The listing builds one solid part. Answer for the finished solid, in the listing's coordinates (mm). Give positions to 0.01 mm unless a question says otherwise; leave off trailing zeros. Order: outer loops, then holes, each group sorted by start corner. A loop starts at its lowest first (then second) coordinate and runs counter-clockwise, first axis right, second up. Notation, with made-up numbers: (-27, 42.25) -> (-12, 42.25) arc R23 cw to (-12, 77.25) -> close; hole circle Ø5 at (74.5, 88). An arc over 180 degrees is marked (long way). Answer as a JSON object with one key per item and string values. Group by question number.
Autodesk Inventor part; units mm, degrees
ref_plane "YZ Plane" through (0, 0, 0) normal (1, 0, 0) x (0, 1, 0)
ref_plane "XZ Plane" through (0, 0, 0) normal (0, 1, 0) x (-1, 0, 0)
ref_plane "XY Plane" through (0, 0, 0) normal (0, 0, 1) x (1, 0, 0)
sketch "Sketch1" plane through (0, 0, 0) normal (0, 0, 1) x (1, 0, 0)
  arc A0 (3.9004, -5.517) -> (1.5898, -4.52) centre (1.5898, -7.6958) ccw
  line L0 (6.8514, -8.6465) -> (3.9004, -5.517)
  arc A1 (6.1121, -10.36) -> (6.8514, -8.6465) centre (6.1121, -9.3437) ccw
  line L1 (-6.1121, -10.36) -> (6.1121, -10.36)
  arc A2 (-6.8514, -8.6465) -> (-6.1121, -10.36) centre (-6.1121, -9.3437) ccw
  line L2 (-3.9004, -5.517) -> (-6.8514, -8.6465)
  arc A3 (-1.5898, -4.52) -> (-3.9004, -5.517) centre (-1.5898, -7.6958) ccw
  line L3 (1.5898, -4.52) -> (-1.5898, -4.52)
  arc A4 (-10.36, -6.3382) -> (-8.5738, -7.0738) centre (-9.3466, -6.4137) ccw
  line L4 (-10.36, 6.3382) -> (-10.36, -6.3382)
  arc A5 (-8.5738, 7.0738) -> (-10.36, 6.3382) centre (-9.3466, 6.4137) ccw
  line L5 (-5.4693, 3.7815) -> (-8.5738, 7.0738)
  arc A6 (-4.38, 1.5898) -> (-5.4693, 3.7815) centre (-7.549, 1.3814) ccw
  line L6 (-4.38, -1.5898) -> (-4.38, 1.5898)
  arc A7 (-5.4693, -3.7815) -> (-4.38, -1.5898) centre (-7.549, -1.3814) ccw
  line L7 (-8.5738, -7.0738) -> (-5.4693, -3.7815)
  arc A8 (8.5693, -7.069) -> (10.36, -6.3423) centre (9.3463, -6.4139) ccw
  line L8 (5.2366, -3.5348) -> (8.5693, -7.069)
  arc A9 (4.38, -1.5898) -> (5.2366, -3.5348) centre (7.5472, -1.356) ccw
  line L9 (4.38, 1.5898) -> (4.38, -1.5898)
  arc A10 (5.2366, 3.5348) -> (4.38, 1.5898) centre (7.5472, 1.356) ccw
  line L10 (8.5693, 7.069) -> (5.2366, 3.5348)
  arc A11 (10.36, 6.3423) -> (8.5693, 7.069) centre (9.3463, 6.4139) ccw
  line L11 (10.36, -6.3423) -> (10.36, 6.3423)
  circle A12 centre (0, 0) radius 2.5
  arc A13 (-4.32, 10.36) -> (-4.32, 12.5) centre (-4.32, 11.43) ccw
  line L12 (-4.32, 12.5) -> (-10.5183, 12.5)
  arc A14 (-10.5183, 12.5) -> (-12.5, 10.5183) centre (-10.5183, 10.5183) ccw
  line L13 (-12.5, 10.5183) -> (-12.5, -10.5215)
  arc A15 (-12.5, -10.5215) -> (-10.6304, -12.5) centre (-10.5183, -10.5215) ccw
  line L14 (-10.6304, -12.5) -> (10.6304, -12.5)
  arc A16 (10.6304, -12.5) -> (12.5, -10.5215) centre (10.5183, -10.5215) ccw
  line L15 (12.5, -10.5215) -> (12.5, 10.5183)
  arc A17 (12.5, 10.5183) -> (10.5183, 12.5) centre (10.5183, 10.5183) ccw
  line L16 (10.5183, 12.5) -> (4.32, 12.5)
  arc A18 (4.32, 12.5) -> (4.32, 10.36) centre (4.32, 11.43) ccw
  line L17 (4.32, 10.36) -> (6.3685, 10.36)
  arc A19 (7.1102, 8.641) -> (6.3685, 10.36) centre (6.3685, 9.3405) ccw
  line L18 (7.1102, 8.641) -> (3.9004, 5.237)
  arc A20 (1.5898, 4.24) -> (3.9004, 5.237) centre (1.5898, 7.4158) ccw
  line L19 (1.5898, 4.24) -> (-1.5898, 4.24)
  arc A21 (-3.9004, 5.237) -> (-1.5898, 4.24) centre (-1.5898, 7.4158) ccw
  line L20 (-3.9004, 5.237) -> (-7.1102, 8.641)
  arc A22 (-6.3685, 10.36) -> (-7.1102, 8.641) centre (-6.3685, 9.3405) ccw
  line L21 (-6.3685, 10.36) -> (-4.32, 10.36)
extrude "Extrusion1" add sketch "Sketch1" against normal blind 100
properties part number "25-2501"
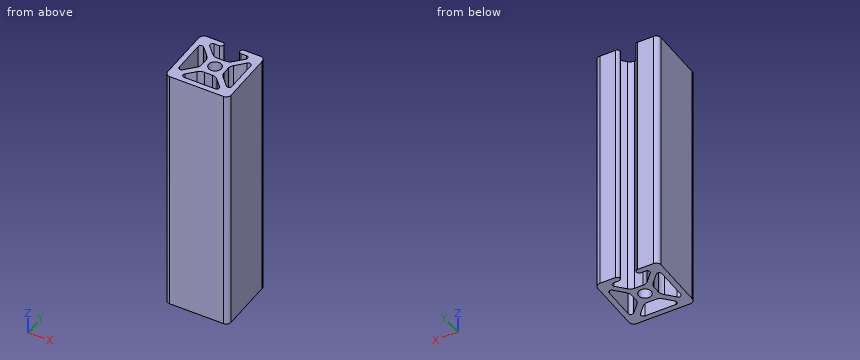
(1) Find the intervals of material crossed by line 1 along Y through (x, z) = (0, -64); line 2 along Y through (x, z) = (-1.25, -85.5); line 3 along X through (y, z) = (-4, -83), in increasing order. Write a range as [from, to].
(2) A cutting plane is placed at C-C (z = -78.5). State how many separate pieces and enclosed holes the cut face has, and give its area (3 significant figures).
(3) A cutting plane is placed at A-A (y = 0). Determine the outline of the cut face in (x, z).
(4) A cutting plane is placed at B-B (x = 0). Determine the outline of the cut face in (y, z).
(5) A flat-ended cylindrical pin translates along its axis: pin 1 Ø2.5 at (x, z) = (-0.5, -49.5) entering from +Y. Find the tip coordinate at first contact, or state that the pin passes through.
(6) A cutting plane is placed at D-D (y = 11.43). Determine the outline of the cut face in (x, z), and give its area (3 significant figures).
Check sheet entries:
{
 "1": {"line 1": "y = [-12.5, -10.36], [-4.52, -2.5], [2.5, 4.24]", "line 2": "y = [-12.5, -10.36], [-4.52, -2.17], [2.17, 4.24]", "line 3": "x = [-12.5, -10.36], [-5.68, 5.68], [10.36, 12.5]"},
 "2": {"separate pieces": "1", "enclosed holes": "4", "area": "322 mm2"},
 "3": {"outline": "(-12.5, -100) -> (-10.36, -100) -> (-10.36, 0) -> (-12.5, 0) -> close; (-4.38, -100) -> (-2.5, -100) -> (-2.5, 0) -> (-4.38, 0) -> close; (2.5, -100) -> (4.38, -100) -> (4.38, 0) -> (2.5, 0) -> close; (10.36, -100) -> (12.5, -100) -> (12.5, 0) -> (10.36, 0) -> close"},
 "4": {"outline": "(-12.5, -100) -> (-10.36, -100) -> (-10.36, 0) -> (-12.5, 0) -> close; (-4.52, -100) -> (-2.5, -100) -> (-2.5, 0) -> (-4.52, 0) -> close; (2.5, -100) -> (4.24, -100) -> (4.24, 0) -> (2.5, 0) -> close"},
 "5": {"pin 1": "stops at y = 4.24"},
 "6": {"outline": "(-12.28, -100) -> (-3.25, -100) -> (-3.25, 0) -> (-12.28, 0) -> close; (3.25, -100) -> (12.28, -100) -> (12.28, 0) -> (3.25, 0) -> close", "area": "1,810 mm2"}
}
